from build123d import *

# Parameters (mm, degrees)
BOSS_EXTRUDE1_DEPTH = 5.002296298
BOSS_EXTRUDE2_REACH = 34.501
BOSS_EXTRUDE3_REACH = 35.167
SKETCH4_W           = 2.497703702
SKETCH4_H           = 2.5
SKETCH5_W           = 2.5
SKETCH5_H           = 2.5
SKETCH6_W           = 2.5
SKETCH6_H           = 2.5
SKETCH7_W           = 2.497703702
SKETCH7_H           = 2.5


with BuildPart() as part:
    # Sketch1 → Boss-Extrude1 (new body)
    with BuildSketch(Plane(origin=(5.002296298, 0, 0), x_dir=(0, 0, -1), z_dir=(1, 0, 0))):
        with BuildLine():
            Line((-5, 0), (-25, 0))
            ThreePointArc((-25, 0), (-30, -5), (-25, -10))
            Line((-25, -10), (-5, -10))
            ThreePointArc((-5, -10), (0, -5), (-5, 0))
        make_face()
    extrude(amount=-BOSS_EXTRUDE1_DEPTH)

    # Sketch2 → Boss-Extrude2 (add, up to next)
    with BuildSketch(Plane(origin=(7.502296298, 0, 0), x_dir=(0, 0, -1), z_dir=(1, 0, 0)), mode=Mode.PRIVATE) as boss_extrude2_sk1:
        with BuildLine():
            Line((-17.5, -2.5), (-17.5, -7.5))
            ThreePointArc((-17.5, -7.5), (-15, -10), (-12.5, -7.5))
            Line((-12.5, -7.5), (-12.5, -2.5))
            ThreePointArc((-12.5, -2.5), (-15, 0), (-17.5, -2.5))
        make_face()
    boss_extrude2_tool1 = extrude(boss_extrude2_sk1.sketch, amount=-BOSS_EXTRUDE2_REACH, mode=Mode.PRIVATE) - part.part
    add(boss_extrude2_tool1.solids().sort_by_distance((7.502296, -5, 15))[0])

    # Sketch3 → Boss-Extrude3 (add, up to next)
    with BuildSketch(Plane(origin=(-2.5, 0, 0), x_dir=(0, -1, 0), z_dir=(-1, 0, 0)), mode=Mode.PRIVATE) as boss_extrude3_sk1:
        with BuildLine():
            Line((7.5, 17.5), (2.5, 17.5))
            ThreePointArc((2.5, 17.5), (0, 15), (2.5, 12.5))
            Line((2.5, 12.5), (7.5, 12.5))
            ThreePointArc((7.5, 12.5), (10, 15), (7.5, 17.5))
        make_face()
    boss_extrude3_tool1 = extrude(boss_extrude3_sk1.sketch, amount=-BOSS_EXTRUDE3_REACH, mode=Mode.PRIVATE) - part.part
    add(boss_extrude3_tool1.solids().sort_by_distance((-2.5, -5, 15))[0])

    # Sketch4 → Revolve1 (revolve)
    with BuildSketch(Plane(origin=(0, 0, 5), x_dir=(-1, 0, 0), z_dir=(0, 0, -1)), mode=Mode.PRIVATE) as revolve1_sk:
        with Locations((1.248851851, -3.75)):
            Rectangle(SKETCH4_W, SKETCH4_H)
    revolve(revolve1_sk.sketch.rotate(Axis((0, -5, 5), (-1, 0, 0)), 270), axis=Axis((0, -5, 5), (-1, 0, 0)))

    # Sketch5 → Revolve2 (revolve)
    with BuildSketch(Plane(origin=(0, 0, 5), x_dir=(-1, 0, 0), z_dir=(0, 0, -1)), mode=Mode.PRIVATE) as revolve2_sk:
        with Locations((-6.252296298, -3.75)):
            Rectangle(SKETCH5_W, SKETCH5_H)
    revolve(revolve2_sk.sketch.rotate(Axis((7.502296298, -5, 5), (-1, 0, 0)), 270), axis=Axis((7.502296298, -5, 5), (-1, 0, 0)))

    # Sketch6 → Revolve3 (revolve)
    with BuildSketch(Plane(origin=(0, 0, 25), x_dir=(-1, 0, 0), z_dir=(0, 0, -1)), mode=Mode.PRIVATE) as revolve3_sk:
        with Locations((-6.252296298, -3.75)):
            Rectangle(SKETCH6_W, SKETCH6_H)
    revolve(revolve3_sk.sketch.rotate(Axis((7.502296298, -5, 25), (-1, 0, 0)), 270), axis=Axis((7.502296298, -5, 25), (-1, 0, 0)))

    # Sketch7 → Revolve4 (revolve)
    with BuildSketch(Plane(origin=(0, 0, 25), x_dir=(-1, 0, 0), z_dir=(0, 0, -1)), mode=Mode.PRIVATE) as revolve4_sk:
        with Locations((1.248851851, -3.75)):
            Rectangle(SKETCH7_W, SKETCH7_H)
    revolve(revolve4_sk.sketch.rotate(Axis((0, -5, 25), (-1, 0, 0)), 270), axis=Axis((0, -5, 25), (-1, 0, 0)))


solid = part.part
The listing builds one solid part. Answer for the finished solid, in the listing's coordinates (mm). A direction names the side the tool comes from. Round coordinates to 2 decimals unless told otherwise and drop trailing zeros. Write each loop counter-clockwise with the first axis right and the second up, starting at its lowest first coordinate (ties: lowest second). Pieces come first, ordered by that corner, then holes. Notation, with made-up numbers: (58, 55) - (81, 55) arc R27 ccw to (81, 82) - close; hole circle Ø8 at (35.5, -3). An arc over 180 degrees is marked (long way). Use one line per item in the form item = value. Start each with the question number.
Item 1: A cutting plane is placed at B-B (z = 23.5). Write down the section's boundary in (x, y).
Item 2: Find the intervals of material crossed by line 1 (Z direction, x = 6.5, y = -4.5); line 2 (Z direction, x = 7.25, y = -6.25); line 3 (X direction, y = -5.75, z = 2.5), in increasing order. Write a range as [from, to].
Item 3: A cutting plane is placed at A-A (x = 6.75). Write down the section's boundary in (y, z), plus the area to 3 significant figures.
Item 4: A tool of negligible diameter and unlimited length cuts with its end or side. For faces 1 (the flat face through (5.002, -3.8, 22.6)), 2 (the flat face through (-1, -5, 17.5)), 3 (the flat face through (6, -5, 17.5)), 4 (the cylindrical face through (-1.27, -3.31, 23.16)), from which of +Z, -Z, +X, -X, +Y, -Y can it reach the whole face along a straight path? Write none if from no direction.
Item 5: Flat-ended cylindrical pins translate along their axes: pin 1 Ø6 at (x, y) = (-0.5, -1) entering from -Z; pin 2 Ø3 at (x, y) = (7, -4.5) entering from -Z; pin 3 Ø5.5 at (y, z) = (-5, 25.5) entering from -X. Find the tip coordinate at first contact, or state that the pin passes through.
Item 6: Determine the mould class of faces 5 (the cylindrical face through (6.23, -3.31, 23.16)), 6 (the cylindrical face through (3, -5, 0)), 7 (the cylindrical face through (-1, -10, 15)) for opening direction Z: +Z half, -Z half, draft (parallel to the pull), parting line (faces both ways), or undercut.
Item 7: A cutting plane is placed at C-C (y = -5). Write down the section's boundary in (x, z).
Item 8: A cutting plane is placed at D-D (x = 1.75). Write down the section's boundary in (y, z), plus the area to 3 significant figures.
The answers:
q1.outline = (-2.5, -7) - (0, -7) - (0, -10) - (5, -10) - (5, -7) - (7.5, -7) - (7.5, -3) - (5, -3) - (5, 0) - (0, 0) - (0, -3) - (-2.5, -3) - close
q2.line_1 = [2.55, 7.45], [12.5, 17.5], [22.55, 27.45]
q2.line_2 = [2.83, 7.17], [12.5, 17.5], [22.83, 27.17]
q2.line_3 = [0, 5]
q3.outline = circle Ø5 at (-5, 5); (-7.5, 12.5) - (-2.5, 12.5) arc R2.5 ccw to (-2.5, 17.5) - (-7.5, 17.5) arc R2.5 ccw to start; circle Ø5 at (-5, 25)
q3.area = 83.9 mm^2
q4.face_1 = +X
q4.face_2 = -X, +Y, -Y
q4.face_3 = +X, +Y, -Y
q4.face_4 = -X
q5.pin_1 = 0.11
q5.pin_2 = 2.5
q5.pin_3 = -2.5
q6.face_5 = undercut
q6.face_6 = -Z half
q6.face_7 = parting line
q7.outline = (-2.5, 2.5) - (0, 2.5) - (0, 0) - (5, 0) - (5, 2.5) - (7.5, 2.5) - (7.5, 7.5) - (5, 7.5) - (5, 12.5) - (7.5, 12.5) - (7.5, 17.5) - (5, 17.5) - (5, 22.5) - (7.5, 22.5) - (7.5, 27.5) - (5, 27.5) - (5, 30) - (0, 30) - (0, 27.5) - (-2.5, 27.5) - (-2.5, 22.5) - (0, 22.5) - (0, 17.5) - (-2.5, 17.5) - (-2.5, 12.5) - (0, 12.5) - (0, 7.5) - (-2.5, 7.5) - close
q8.outline = (-10, 5) arc R5 ccw to (0, 5) - (0, 25) arc R5 ccw to (-10, 25) - close
q8.area = 279 mm^2
